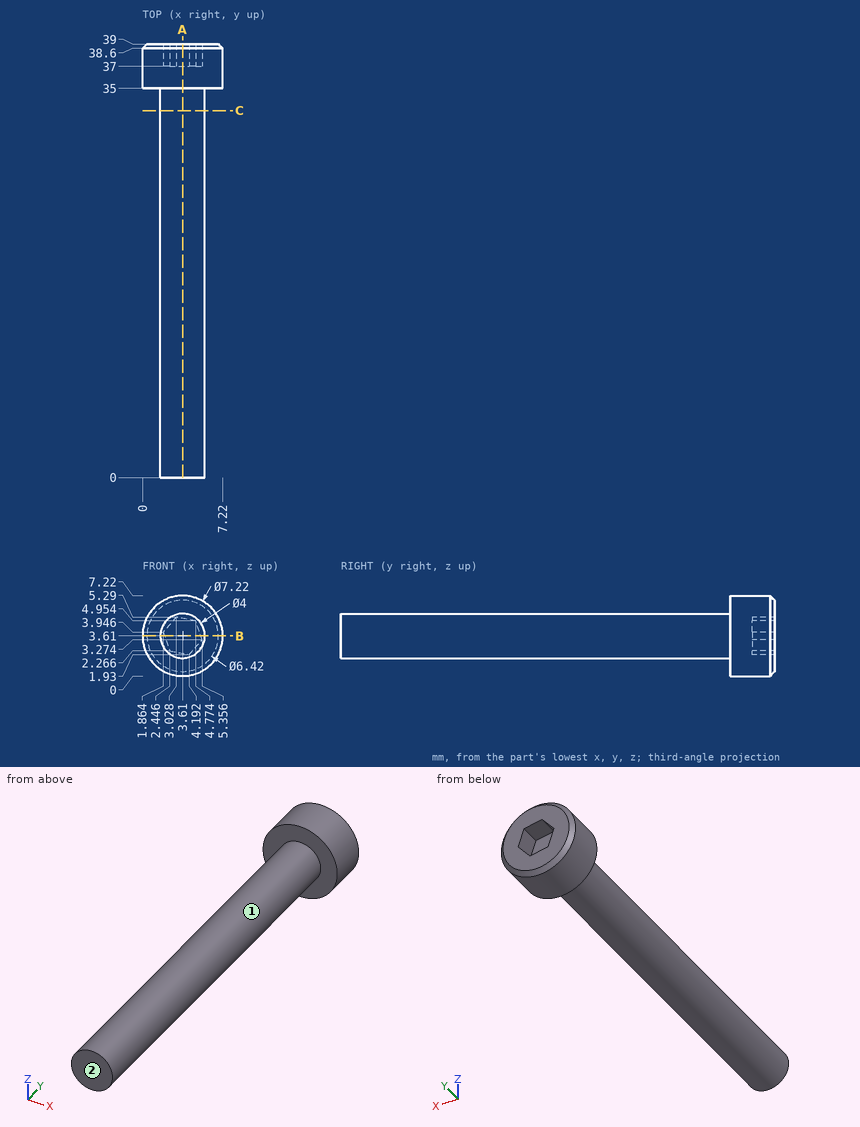
Part print with two shaded views. Sizes in mm from the minimum x, y, z corner. A direction names the side the tool comes from. Round coordinates to 2 decimals unless told otherwise and drop trailing zeros. Order: outer loops, then holes, each group sorted by start corner. A loop starts at its lowest first (then second) coordinate and runs counter-clockwise, first axis right, second up. Notation, with made-up numbers: (22, 45.25) -> (81, 45.25) arc R27 ccw to (81, 81.25) -> close; hole circle Ø1 at (41, 31). An arc over 180 degrees is marked (long way). Use one line per item in the form item = value.
Item 1: Drill centre lines: line 1 (Y direction, x = 2.75, z = 4); line 2 (Y direction, x = 1.5, z = 3.25); line 3 (Z direction, x = 4.75, y = 11). Where is each one in solid material? Low to high.
Returned:
line_1 = 0 to 37
line_2 = 35 to 39
line_3 = 1.97 to 5.25
Item 2: Cut at B-B, the plane z = 3.61. Write the cut outline in (x, y).
Returned:
outline = (0, 35) -> (1.61, 35) -> (1.61, 0) -> (5.61, 0) -> (5.61, 35) -> (7.22, 35) -> (7.22, 38.6) -> (6.82, 39) -> (5.24, 39) -> (5.24, 37) -> (1.98, 37) -> (1.98, 39) -> (0.4, 39) -> (0, 38.6) -> close
Item 3: Cut at A-A, the plane x = 3.61. Write the cut outline in (y, z).
Returned:
outline = (0, 1.61) -> (35, 1.61) -> (35, 0) -> (38.6, 0) -> (39, 0.4) -> (39, 2.04) -> (37, 2.04) -> (37, 5.18) -> (39, 5.18) -> (39, 6.82) -> (38.6, 7.22) -> (35, 7.22) -> (35, 5.61) -> (0, 5.61) -> close
Item 4: Flat gauge pins, fed straight in: pin 1 Ø2.5 at (x, z) = (3.5, 3.5) entering from +Y; pin 2 Ø2 at (y, z) = (10, 6) entering from -X; pin 3 Ø2 at (x, y) = (2.5, 16.5) entering from +Z. Where does each tip first touch, or does it go through?
Returned:
pin_1 = 37
pin_2 = 2.17
pin_3 = 5.61
Item 5: Tool access for the marked faces 1 and 2: list every direction of +Z, -Z, +X, -X, +Y, -Y with a clear straight run to the whole face (end or side of a thin tool).
Returned:
face_1 = -Y
face_2 = +Z, -Z, +X, -X, -Y
Item 6: Cut at C-C, the plane y = 33. Write the cut outline in (x, z).
Returned:
outline = circle Ø4 at (3.61, 3.61)
